Source: CAD feature listing. Evaluate the final solid. Frame: model axes, mm. A direction names the side the tool comes from. Give positions to 0.01 mm unless a question says otherwise; leave off trailing zeros. Order: outer loops, then holes, each group sorted by start corner. A loop starts at its lowest first (then second) coordinate and runs counter-clockwise, first axis right, second up.
Autodesk Inventor part; units mm, degrees
ref_plane "YZ Plane" through (0, 0, 0) normal (1, 0, 0) x (0, 1, 0)
ref_plane "XZ Plane" through (0, 0, 0) normal (0, 1, 0) x (-1, 0, 0)
ref_plane "XY Plane" through (0, 0, 0) normal (0, 0, 1) x (1, 0, 0)
sketch "Sketch1" plane through (0, 0, 0) normal (0, 1, 0) x (-1, 0, 0)
  line L0 (0, 0) -> (72.9, 0)
  line L1 (72.9, 0) -> (72.9, -61.3)
  line L2 (72.9, -61.3) -> (0, -61.3)
  line L3 (0, -61.3) -> (0, 0)
  dimension "d0" = 72.9
  dimension "d1" = 61.3
extrude "Extrusion1" add sketch "Sketch1" along normal blind 2.5
sketch "Sketch2" plane through (0, 2.5, 0) normal (0, 1, 0) x (1, 0, 0)
  line L0 (-72.9, 0) -> (0, 0)
  line L1 (-72.9, 61.3) -> (-72.9, 0)
  line L2 (0, 61.3) -> (-72.9, 61.3)
  line L3 (0, 0) -> (0, 61.3)
  point P0 (-65.2, 53.8)
  point P1 (-7.8, 7.5)
  dimension "d6" = 7.7
  dimension "d7" = 7.5
  dimension "d8" = 7.5
  dimension "d9" = 7.8
hole "Hole1" at (-65.2, 2.5, -53.8) at (-7.8, 2.5, -7.5) direction (0, -1, 0) diameter 4 end through all
sketch "Sketch3" plane through (0, 2.5, 0) normal (0, 1, 0) x (1, 0, 0)
  line L0 (-57.9, 38.9915) -> (-15.0143, 38.9915) construction
  line L1 (-15.0143, 38.9915) -> (-15.0143, 22.3) construction
  line L2 (-15.0143, 22.3) -> (-57.9, 22.3) construction
  line L3 (-57.9, 22.3) -> (-57.9, 38.9915) construction
  line L4 (-72.9, 61.3) -> (-72.9, 0)
  line L5 (-72.9, 0) -> (0, 0)
  spline S0 degree 2 poles (-52.0066, 22.2116) (-54.2985, 22.2116) (-56.7541, 24.9537) (-56.7677, 27.6003) knots 0 0 0 1 2 2 2
  line L6 (-56.7677, 27.6003) -> (-56.7677, 29.0873)
  spline S1 degree 2 poles (-56.7677, 29.0873) (-56.7677, 31.843) (-54.3803, 34.9671) (-52.2248, 34.9671) knots 0 0 0 1 2 2 2
  spline S2 degree 2 poles (-52.2248, 34.9671) (-50.0694, 34.9671) (-47.9275, 32.2114) (-47.9139, 29.3056) knots 0 0 0 1 2 2 2
  line L7 (-47.9139, 29.3056) -> (-47.9139, 27.9823)
  line L8 (-47.9139, 27.9823) -> (-54.7759, 27.9823)
  line L9 (-54.7759, 27.9823) -> (-54.7759, 27.6958)
  spline S3 degree 2 poles (-54.7759, 27.6958) (-54.7759, 25.7177) (-53.2889, 23.9305) (-51.8838, 23.9305) knots 0 0 0 1 2 2 2
  spline S4 degree 2 poles (-51.8838, 23.9305) (-50.997, 23.9305) (-49.6465, 24.599) (-49.0598, 25.3221) knots 0 0 0 1 2 2 2
  line L10 (-49.0598, 25.3221) -> (-48.0094, 24.0533)
  spline S5 degree 2 poles (-48.0094, 24.0533) (-49.319, 22.2116) (-52.0066, 22.2116) knots 0 0 0 1 1 1
  spline S6 degree 2 poles (-52.2248, 33.2345) (-53.4799, 33.2345) (-54.6804, 31.5156) (-54.7623, 29.7148) knots 0 0 0 1 2 2 2
  line L11 (-54.7623, 29.7148) -> (-49.9193, 29.7148)
  line L12 (-49.9193, 29.7148) -> (-49.9193, 29.9877)
  spline S7 degree 2 poles (-49.9193, 29.9877) (-50.0012, 31.7339) (-51.1062, 33.2345) (-52.2248, 33.2345) knots 0 0 0 1 2 2 2
  line L13 (-34.3808, 22.4435) -> (-36.4817, 22.4435)
  line L14 (-36.4817, 22.4435) -> (-36.4817, 30.0832)
  line L15 (-36.4817, 30.0832) -> (-43.1391, 30.0832)
  line L16 (-43.1391, 30.0832) -> (-43.1391, 22.4435)
  line L17 (-43.1391, 22.4435) -> (-45.2127, 22.4435)
  line L18 (-45.2127, 22.4435) -> (-45.2127, 38.9915)
  line L19 (-45.2127, 38.9915) -> (-43.1391, 38.9915)
  line L20 (-43.1391, 38.9915) -> (-43.1391, 31.8703)
  line L21 (-43.1391, 31.8703) -> (-36.4817, 31.8703)
  line L22 (-36.4817, 31.8703) -> (-36.4817, 38.9915)
  line L23 (-36.4817, 38.9915) -> (-34.3808, 38.9915)
  line L24 (-34.3808, 38.9915) -> (-34.3808, 22.4435)
  line L25 (-28.6102, 22.4435) -> (-30.6974, 22.4435)
  line L26 (-30.6974, 22.4435) -> (-30.6974, 38.9915)
  line L27 (-30.6974, 38.9915) -> (-28.6102, 38.9915)
  line L28 (-28.6102, 38.9915) -> (-28.6102, 22.4435)
  line L29 (-15.2817, 37.2044) -> (-19.6336, 37.2044)
  line L30 (-19.6336, 37.2044) -> (-19.6336, 22.4435)
  line L31 (-19.6336, 22.4435) -> (-21.7209, 22.4435)
  line L32 (-21.7209, 22.4435) -> (-21.7209, 37.2044)
  line L33 (-21.7209, 37.2044) -> (-26.0591, 37.2044)
  line L34 (-26.0591, 37.2044) -> (-26.0591, 38.9915)
  line L35 (-26.0591, 38.9915) -> (-15.2817, 38.9915)
  line L36 (-15.2817, 38.9915) -> (-15.2817, 37.2044)
  dimension "d17" = 42.8857
  dimension "d18" = 15
  dimension "d19" = 16.6915
  dimension "d20" = 22.3
extrude "Extrusion2" add sketch "Sketch3" along normal blind 2
properties part number "Lid"
1) Section query A-A, the plane z = -7.5. Return the cut outline in (x, y), and give its area (3 significant figures).
Report:
outline: (-72.9, 0) - (-9.8, 0) - (-9.8, 2.5) - (-72.9, 2.5) - close; (-5.8, 0) - (0, 0) - (0, 2.5) - (-5.8, 2.5) - close
area: 172 mm2
2) Section query B-B, the plane x = -7.8. Return the cut outline in (y, z).
Report:
outline: (0, -61.3) - (2.5, -61.3) - (2.5, -9.5) - (0, -9.5) - close; (0, -5.5) - (2.5, -5.5) - (2.5, 0) - (0, 0) - close
3) Material intervals for L1, parallel to X at y = 3.1, z = -28.5; L2, parallel to Z at x = -7.8, y = 0.6; L3, parallel to X at y = 3.95, z = -24.5 (3 decimals), sorted ascending.
Report:
L1: x = -56.77 to -47.91, -45.21 to -43.14, -36.48 to -34.38, -30.7 to -28.61, -21.72 to -19.63
L2: z = -61.3 to -9.5, -5.5 to 0
L3: x = -56.144 to -53.706, -49.925 to -48.379, -45.213 to -43.139, -36.482 to -34.381, -30.697 to -28.61, -21.721 to -19.634
4) Pin query (flat end, axial travel): pin 1 (1 mm diameter, centred on x = -38.5, y = 4, fed in from +Z); pin 2 (0.6 mm diameter, centred on x = -44, y = 3, fed in from -Z); pin 3 (1 mm diameter, centred on y = 3.5, z = -34, fed in from +X); pin 4 (5 mm diameter, centred on x = -31, z = -39.5, fed in from -Y). Return the tip coordinate at first contact, or that it passes through.
Report:
pin 1: stops at z = -30.08
pin 2: stops at z = -38.99
pin 3: stops at x = -19.63
pin 4: stops at y = 0
5) Reachability of faces 1 (the flat face through (-40, 3, -31.87)), 2 (the flat face through (-35, 3, -22.444)), 3 (the flat face through (-51, 3, -27.982)), 4 (the flat face through (-34.381, 3, -31)), 5 (the flat face through (-24, 3, -37.204)) from +Z, -Z, +X, -X, +Y, -Y: full face, straight path, thin tool, end or side. Return the list, or none.
Report:
face 1: -Z, +Y
face 2: +Z, +X, +Y
face 3: +Y
face 4: +Z, -Z, +Y
face 5: +Z, +Y
6) Draft query along X for faces 6 (the flat face through (-72.9, 1, -30)), 7 (the flat face through (-28.61, 3, -31)), 8 (the flat face through (-30, 3, -38.992)). Return one class per face: +X half, -X half, draft (parallel to the pull), parting line (faces both ways), or undercut.
Report:
face 6: -X half
face 7: undercut
face 8: draft
7) Section query C-C, the plane y = 3.3. Count the separate pieces of the cut face and the enclosed holes in it, and give its area (3 significant figures).
Report:
separate pieces: 4
enclosed holes: 1
area: 225 mm2
